Verification items for this drawing (mm, ordinates from the low corner). Round coordinates to 2 decimals unless told otherwise and drop trailing zeros. Loops run counter-clockwise (first coordinate to the right, second up) from the corner with the lowest first, then second, coordinate; pieces in that order, holes last. Notation, with made-up numbers: (48, -31.5) - (94, -31.5) arc R22 cw to (94, -20.5) - close; hole circle Ø2 at (6.5, -33.5). An arc over 180 degrees is marked (long way). Put each result on its own line as item: value. Start each with the question number.
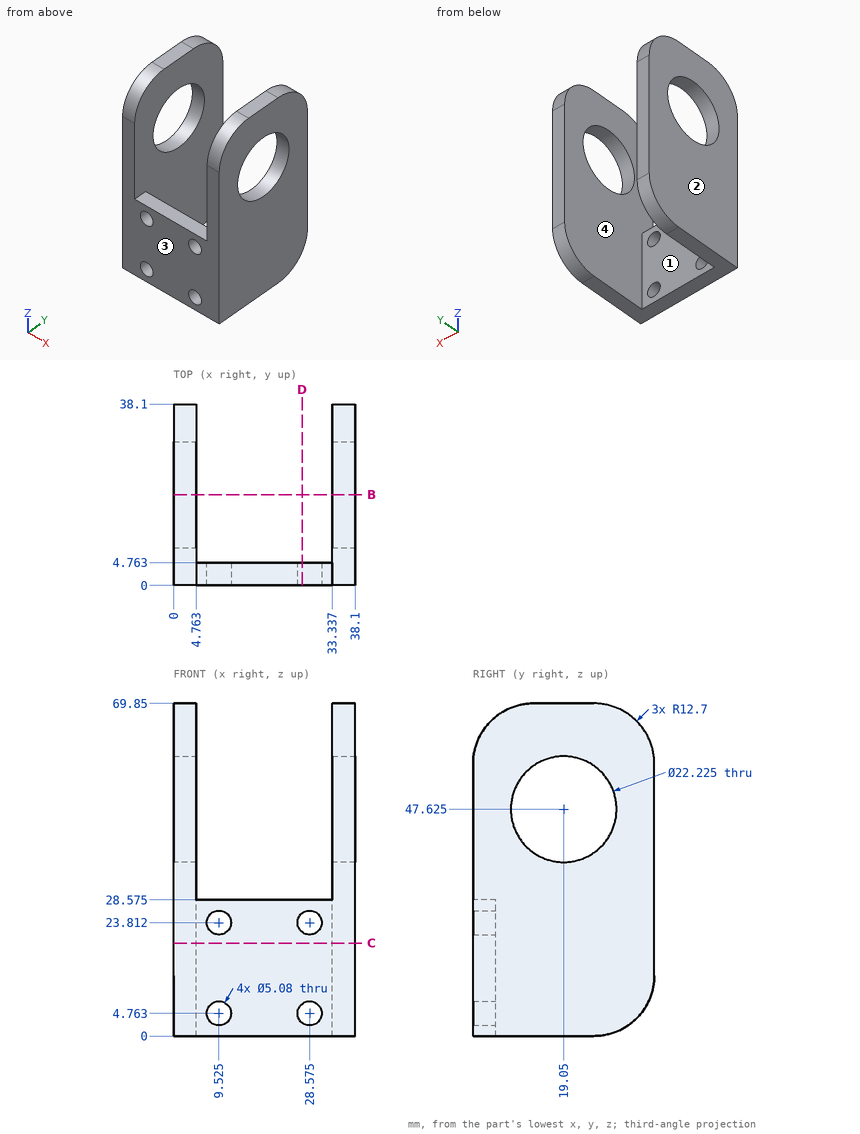
Q1. Depth check by flat-ended pin: pin 1 Ø11.5 at (y, z) = (27.5, 41) entering from +X; pin 2 Ø4.5 at (x, z) = (28.58, 4.76) entering from -Y; pin 3 Ø10 at (x, y) = (23, 9.5) entering from +Z (1 decimal); pin 4 Ø8 at (x, z) = (9.52, 4.76) entering from +Y. Enter the tip coordinate at first touch or a pass-through.
Q2. Cross-section at B-B on y = 19.05. Enter the section's corners in (x, z).
Q3. Material ranges on line 1 (Z direction, x = 36.5, y = 19.5); line 2 (X direction, y = 10, z = 21); line 3 (Y direction, x = 12, z = 11), recorded low to high. Write a range as from..to.
Q4. Cross-section at C-C on z = 19.5. Enter the section's corners in (x, y).
Q5. Draft check along X on the marked faces 1, 2, 3 and 4. Enter one of: +X half, -X half, draft (parallel to the pull), parting line (faces both ways), or undercut.
Q6. Cross-section at D-D on x = 27. Enter the section's corners in (y, z) (1 decimal).
Answer list:
1. pin 1: stops at x = 38.1
1. pin 2: passes through
1. pin 3: stops at z = 28.6
1. pin 4: stops at y = 4.76
2. outline: (0, 0) - (4.76, 0) - (4.76, 36.51) - (0, 36.51) - close; (0, 58.74) - (4.76, 58.74) - (4.76, 69.85) - (0, 69.85) - close; (33.34, 0) - (38.1, 0) - (38.1, 36.51) - (33.34, 36.51) - close; (33.34, 58.74) - (38.1, 58.74) - (38.1, 69.85) - (33.34, 69.85) - close
3. line 1: z = 0..36.52, 58.73..69.85
3. line 2: x = 0..4.76, 33.34..38.1
3. line 3: y = 0..4.76
4. outline: (0, 0) - (38.1, 0) - (38.1, 38.1) - (33.34, 38.1) - (33.34, 4.76) - (4.76, 4.76) - (4.76, 38.1) - (0, 38.1) - close
5. face 1: undercut
5. face 2: -X half
5. face 3: draft
5. face 4: undercut
6. outline: (0, 0) - (4.8, 0) - (4.8, 2.8) - (0, 2.8) - close; (0, 6.8) - (4.8, 6.8) - (4.8, 21.8) - (0, 21.8) - close; (0, 25.8) - (4.8, 25.8) - (4.8, 28.6) - (0, 28.6) - close
